Could you check a few things on this model? Use its own coordinates, in mm. A direction names the side the tool comes from. Give positions to 0.01 mm unless a question says otherwise; leave off trailing zeros. Loops run counter-clockwise (first coordinate to the right, second up) from the corner with the lowest first, then second, coordinate; pieces in that order, holes last. Notation, with made-up numbers: M 81,43.5 L 110,43.5 A21 cw 110,61.5 Z; hole C -33.5,40 d11. An arc over 180 degrees is marked long. Use CSV: the item, a comma, the result in double quotes.
```python
from build123d import *

# Parameters (mm, degrees)
CROQUIS2_W              = 300
CROQUIS2_H              = 180
SALIENTE_EXTRUIR3_DEPTH = 70
CROQUIS3_W              = 40
CROQUIS3_H              = 70
CORTAR_EXTRUIR1_DEPTH   = 70
CROQUIS4_R              = 7.5
CORTAR_EXTRUIR2_DEPTH   = 400
REDONDEO2_R             = 5
REDONDEO3_R             = 5
REDONDEO4_R             = 5
REDONDEO5_R             = 5
REDONDEO6_R             = 5
REDONDEO7_R             = 5
REDONDEO8_R             = 5
REDONDEO9_R             = 5


with BuildPart() as part:
    # Croquis2 → Saliente-Extruir3 (new body)
    with BuildSketch(Plane.XY):
        with Locations((150, 90)):
            Rectangle(CROQUIS2_W, CROQUIS2_H)
    extrude(amount=SALIENTE_EXTRUIR3_DEPTH)

    # Croquis3 → Cortar-Extruir1 (cut)
    with BuildSketch(Plane.XY.offset(70)):
        with Locations((30, 145)):
            Rectangle(CROQUIS3_W, CROQUIS3_H)
        with Locations((270, 35)):
            Rectangle(CROQUIS3_W, CROQUIS3_H)
        with Locations((30, 35)):
            Rectangle(CROQUIS3_W, CROQUIS3_H)
        with Locations((270, 145)):
            Rectangle(CROQUIS3_W, CROQUIS3_H)
    extrude(amount=-CORTAR_EXTRUIR1_DEPTH, mode=Mode.SUBTRACT)

    # Croquis4 → Cortar-Extruir2 (cut)
    with BuildSketch(Plane(origin=(300, 0, 0), x_dir=(0, 0, -1), z_dir=(1, 0, 0))):
        with Locations((-52.5, 157.5)):
            Circle(CROQUIS4_R)
        with Locations((-52.5, 22.5)):
            Circle(CROQUIS4_R)
    extrude(amount=-CORTAR_EXTRUIR2_DEPTH, mode=Mode.SUBTRACT)

    # Redondeo2
    redondeo2_edges = [part.edges().sort_by_distance(p)[0] for p in [
        (150, 0, 70),
    ]]
    fillet(redondeo2_edges, radius=REDONDEO2_R)

    # Redondeo3
    redondeo3_edges = [part.edges().sort_by_distance(p)[0] for p in [
        (150, 180, 70),
    ]]
    fillet(redondeo3_edges, radius=REDONDEO3_R)

    # Redondeo4
    redondeo4_edges = [part.edges().sort_by_distance(p)[0] for p in [
        (5, 180, 70),
    ]]
    fillet(redondeo4_edges, radius=REDONDEO4_R)

    # Redondeo5
    redondeo5_edges = [part.edges().sort_by_distance(p)[0] for p in [
        (295, 180, 70),
    ]]
    fillet(redondeo5_edges, radius=REDONDEO5_R)

    # Redondeo6
    redondeo6_edges = [part.edges().sort_by_distance(p)[0] for p in [
        (295, 0, 70),
    ]]
    fillet(redondeo6_edges, radius=REDONDEO6_R)

    # Redondeo7
    redondeo7_edges = [part.edges().sort_by_distance(p)[0] for p in [
        (5, 0, 70),
    ]]
    fillet(redondeo7_edges, radius=REDONDEO7_R)

    # Redondeo8
    redondeo8_edges = [part.edges().sort_by_distance(p)[0] for p in [
        (0, 90, 70),
        (0, 180, 32.5),
        (0, 0, 32.5),
    ]]
    fillet(redondeo8_edges, radius=REDONDEO8_R)

    # Redondeo9
    redondeo9_edges = [part.edges().sort_by_distance(p)[0] for p in [
        (300, 180, 32.5),
        (300, 90, 70),
        (300, 0, 32.5),
    ]]
    fillet(redondeo9_edges, radius=REDONDEO9_R)


solid = part.part
```
1. Which directions (+Z, -Z, +X, -X, +Y, -Y) give clear straight access to the entire face, cutting with the end or side of a thin tool? Please do faces 4 (the face through (270, 110, 35)), 5 (the face through (300, 89, 32)), 6 (the face through (270, 70, 35)).
Outcome:
face 4,"+Z, -Z, +Y"
face 5,"+Z, -Z, +X, +Y, -Y"
face 6,"+Z, -Z, -Y"
2. I want a section at C-C, the plane z = 10. List the corners of the cut face in (x, y) for me, then the cut area to 3 significant figures.
Outcome:
outline,"M 0,5 A5 ccw 5,0 L 10,0 L 10,70 L 50,70 L 50,0 L 250,0 L 250,70 L 290,70 L 290,0 L 295,0 A5 ccw 300,5 L 300,175 A5 ccw 295,180 L 290,180 L 290,110 L 250,110 L 250,180 L 50,180 L 50,110 L 10,110 L 10,180 L 5,180 A5 ccw 0,175 Z"
area,"42,800 mm2"
3. I want a section at A-A, the plane y = 157.5. List the corners of the cut face in (x, z) for me.
Outcome:
outline,"M 0,0 L 10,0 L 10,45 L 0,45 Z; M 0,60 L 10,60 L 10,70 L 5,70 A5 ccw 0,65 Z; M 50,0 L 250,0 L 250,45 L 50,45 Z; M 50,60 L 250,60 L 250,70 L 50,70 Z; M 290,0 L 300,0 L 300,45 L 290,45 Z; M 290,60 L 300,60 L 300,65 A5 ccw 295,70 L 290,70 Z"
4. I want a section at B-B, the plane x = 142. List the corners of the cut face in (y, z) for me, then the cut area to 3 significant figures.
Outcome:
outline,"M 0,0 L 180,0 L 180,65 A5 ccw 175,70 L 5,70 A5 ccw 0,65 Z; hole C 22.5,52.5 d15; hole C 157.5,52.5 d15"
area,"12,200 mm2"
5. Please list where these lines run through material, in increasing order: line 1 (X direction, y = 28, z = 40.5); line 2 (Z direction, x = 203, y = 157); line 3 (Y direction, x = 5, z = 52.5).
Outcome:
line 1,"0 to 10, 50 to 250, 290 to 300"
line 2,"0 to 45.02, 59.98 to 70"
line 3,"0 to 15, 30 to 150, 165 to 180"
6. I'm going to push a flat-ended pin straight in: pin 1 Ø20 at (x, z) = (265.5, 39.5) entering from -Y. Where does the tip first touch, or does it pass through?
Outcome:
pin 1,"y = 70"
7. If we mould it in two halves opening along Y, with no side actions, what happens to faces 1 (the face through (10, 145, 35)), 2 (the face through (149, 0, 32)), 3 (the face through (151.4, 164.936, 53.476))? For each: +Y half, -Y half, draft (parallel to the pull), parting line (faces both ways), or undercut.
Outcome:
face 1,"draft"
face 2,"-Y half"
face 3,"undercut"
8. I want a section at D-D, the plane x = 265.5. List the corners of the cut face in (y, z) for me.
Outcome:
outline,"M 70,0 L 110,0 L 110,70 L 70,70 Z"
